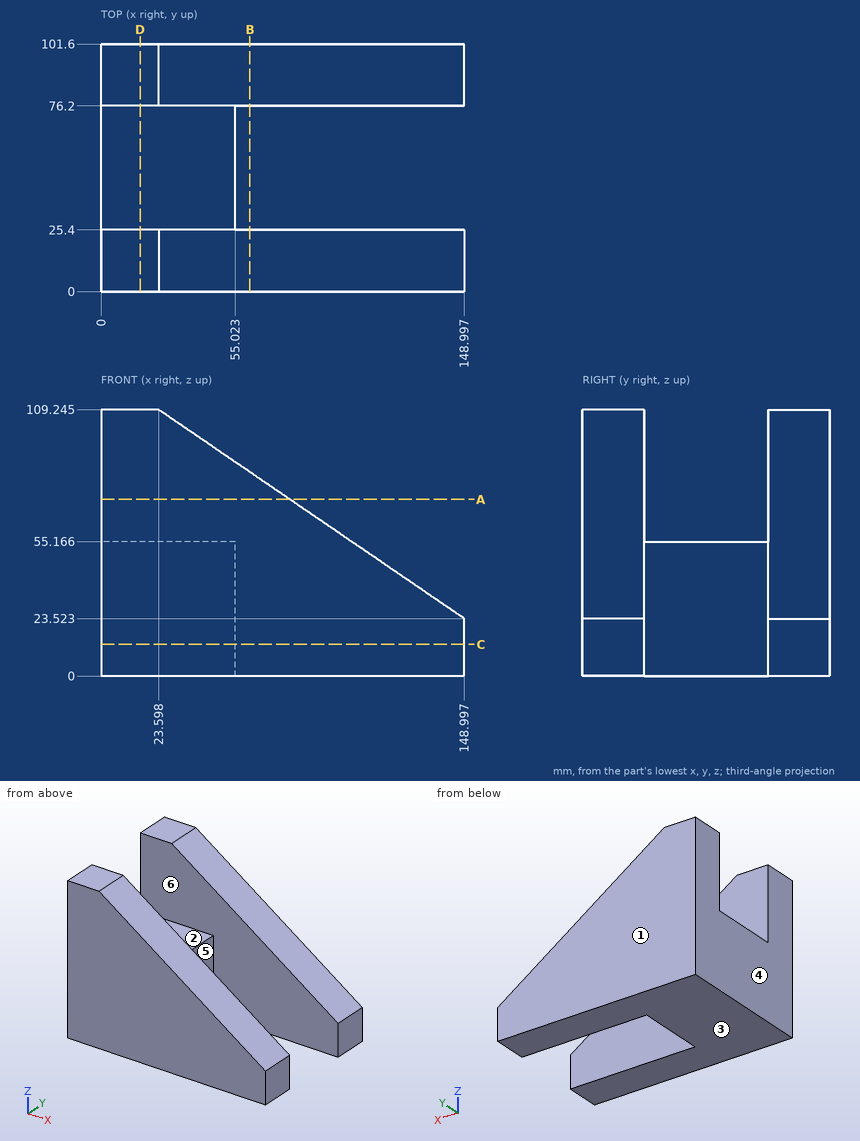
For this review, use the dimensioned drawing (mm, ordinates from the lowest corner) and the shaded views. A direction names the side the tool comes from. Coordinates: 2 decimals unless noted, no trailing zeros. Loops run counter-clockwise (first coordinate to the right, second up) from the corner with the lowest first, then second, coordinate; pieces in that order, holes last.
1. Mouldability with a two-part tool opening along Y and no side actions: class the marked faces 1, 2 and 3 as +Y half, -Y half, draft (parallel to the pull), parting line (faces both ways), or undercut.
2. Add section C-C, the plane z = 13. Give the boundary of the cut face in (x, y).
3. Insertion check: P1, Ø4, axis at x = 98.5, y = 17, coming from the +Z side; P2, Ø3, axis at x = 29, y = 63.5, coming from the +Z side. Each pin has a flat end and moves straight along its axis. Give the tip position at first contact, or say it passes through.
4. Add section A-A, the plane z = 72.5. Give the boundary of the cut face in (x, y).
5. For line 1 (Y direction, x = 69.5, z = 35.5); line 2 (X direction, y = 34.5, z = 55); line 3 (Z direction, x = 14, y = 48) (1 decimal), list the stretches that pass through material, from the lowest coordinate up.
6. For the marked faces 4, 5 and 6, list the 3-axis set-ups (+Z, -Z, +X, -X, +Y, -Y) from which the entire face can be reached by the end or side of a thin tool; tool diameter is ignored.
7. Add section B-B, the plane x = 61. Give the boundary of the cut face in (y, z).
8. Add section D-D, the plane x = 16. Give the boundary of the cut face in (y, z) (1 decimal), then the cut area to 3 significant figures.
Result:
1. face 1: +Y half
1. face 2: undercut
1. face 3: draft
2. outline: (0, 0) - (149, 0) - (149, 25.4) - (55.02, 25.4) - (55.02, 76.2) - (149, 76.2) - (149, 101.6) - (0, 101.6) - close
3. P1: stops at z = 59.41
3. P2: stops at z = 55.17
4. outline: (0, 0) - (77.35, 0) - (77.35, 25.4) - (0, 25.4) - close; (0, 76.2) - (77.35, 76.2) - (77.35, 101.6) - (0, 101.6) - close
5. line 1: y = 0 to 25.4, 76.2 to 101.6
5. line 2: x = 0 to 55.02
5. line 3: z = 0 to 55.2
6. face 4: +Z, -Z, -X, +Y, -Y
6. face 5: +Z, -Z, +X
6. face 6: +Z, +X
7. outline: (0, 0) - (25.4, 0) - (25.4, 83.68) - (0, 83.68) - close; (76.2, 0) - (101.6, 0) - (101.6, 83.68) - (76.2, 83.68) - close
8. outline: (0, 0) - (101.6, 0) - (101.6, 109.2) - (76.2, 109.2) - (76.2, 55.2) - (25.4, 55.2) - (25.4, 109.2) - (0, 109.2) - close
8. area: 8,350 mm2
